Could you check a few things on this drawing? It's one solid part, dimensions in mm from its lowest x, y, z. Coordinates: 2 decimals unless noted, no trailing zeros. Order: outer loops, then holes, each group sorted by start corner. A loop starts at its lowest first (then second) coordinate and runs counter-clockwise, first axis right, second up. Notation, with made-up numbers: M -31.5,64.25 L 26.5,64.25 A24 ccw 26.5,99.25 Z; hole C 11,-21 d3. An arc over 180 degrees is marked long. Answer as CSV lines item,"result". Start each with the question number.
1. If we section it at A-A (z = 87.5): List the corners of the cut face in (x, y) for me.
2. If we section it at C-C (x = 30.5): List the corners of the cut face in (y, z) for me.
3. If we section it at B-B (y = 2.2): Give the number of separate pieces and of enclosed holes in the cut face, plus the area to 3 significant figures.
4. I need wall thicknesses on line 1 along Z through (x, y) = (25, 2.3); line 2 along Z through (x, y) = (86.5, 2.35). Which ranges of each line are inside material? Lowest first, please. Write a range as from..to.
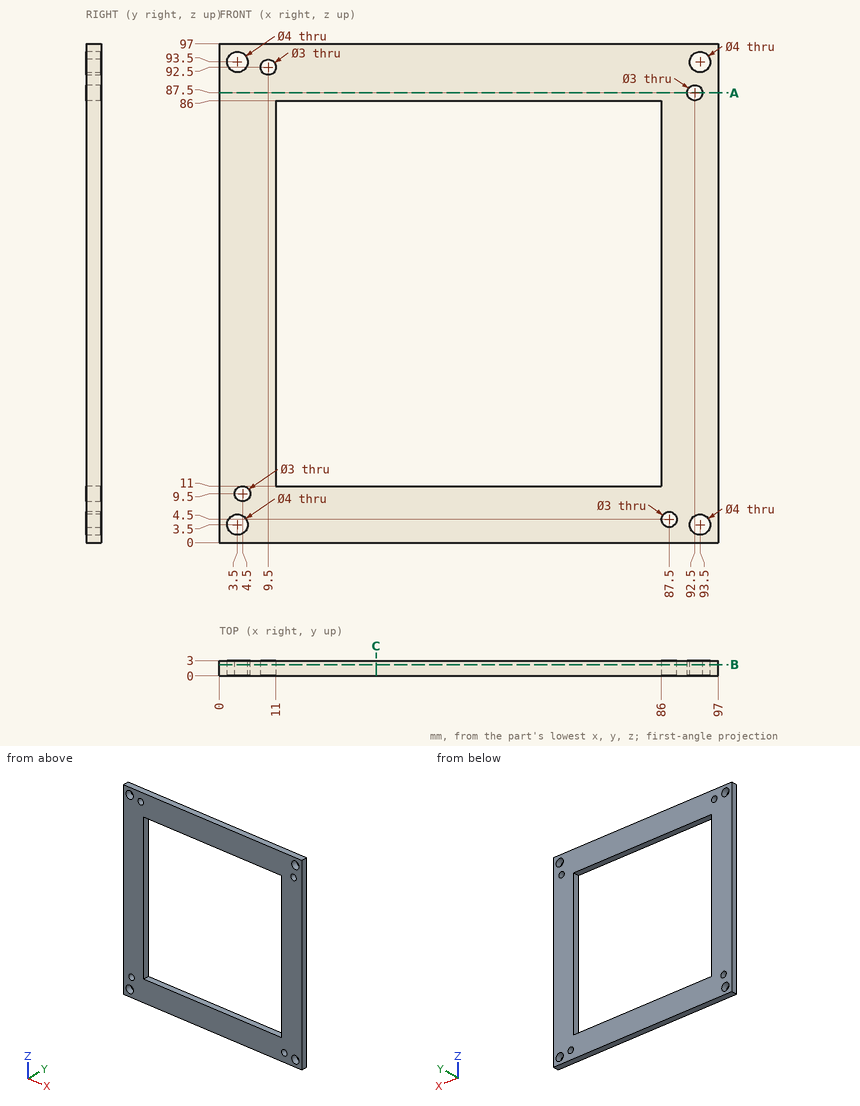
Solved:
1,outline,"M 0,0 L 91,0 L 91,3 L 0,3 Z; M 94,0 L 97,0 L 97,3 L 94,3 Z"
2,outline,"M 0,0 L 3,0 L 3,11 L 0,11 Z; M 0,86 L 3,86 L 3,97 L 0,97 Z"
3,separate pieces,"1"
3,enclosed holes,"9"
3,area,"3,710 mm²"
4,line 1,"0..11, 86..97"
4,line 2,"0..3.38, 5.62..97"
